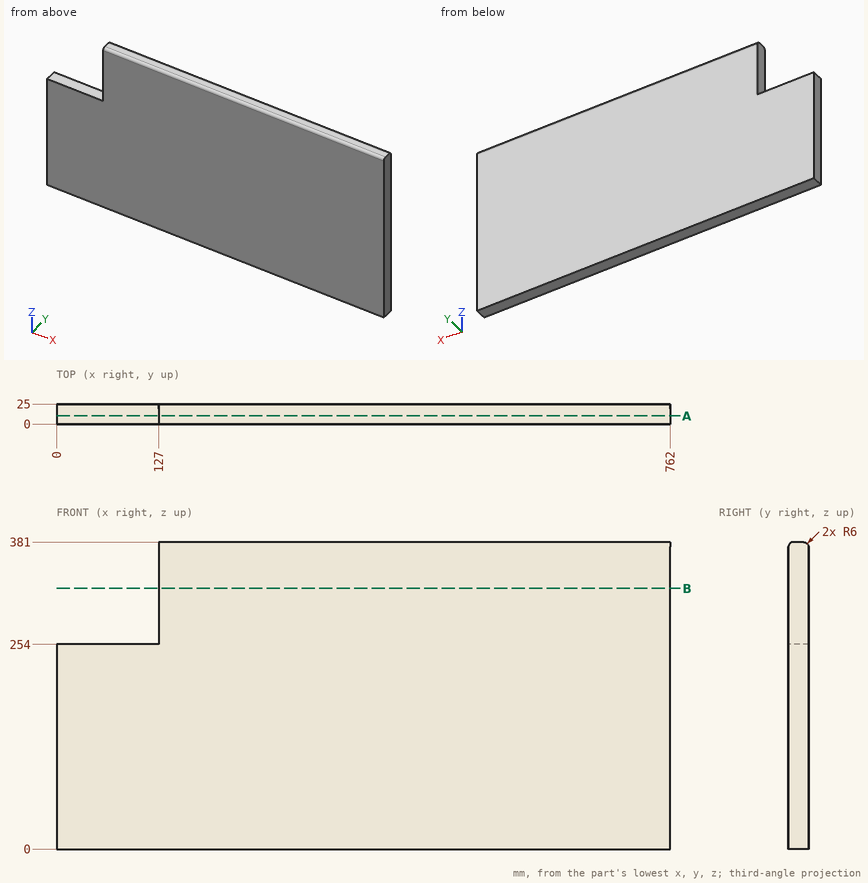
The drawing under review shows one solid part. Ordinate dimensions are in mm from its lowest x, y, z. Give positions to 0.01 mm unless a question says otherwise; leave off trailing zeros. Order: outer loops, then holes, each group sorted by start corner. A loop starts at its lowest first (then second) coordinate and runs counter-clockwise, first axis right, second up. Notation, with made-up numbers: (23.5, -1) -> (53.5, -1) arc R16 cw to (53.5, 10) -> close; hole circle Ø6 at (74.5, -20). An arc over 180 degrees is marked (long way). Write item = value, one per line.
1) Insertion check: pin 1 (12.5 mm diameter, centred on y = 10.5, z = 337.5, fed in from -X). The pin has a flat end and moves straight along its axis. Give the tip position at first contact, or say it passes through.
Findings:
pin_1 = 127
2) We need section B-B, the plane z = 323.5. Give the boundary of the cut face in (x, y), and give its area (3 significant figures).
Findings:
outline = (127, 0) -> (762, 0) -> (762, 25) -> (127, 25) -> close
area = 15,900 mm^2
3) To check wall thickness, follow L1, parallel to Z at x = 65, y = 20.75; L2, parallel to X at y = 21.75, z = 265; L3, parallel to Z at x = 513.5, y = 5.5. State the ranges of each line that lie inside material, in increasing order. Write a range as from..to.
Findings:
L1 = 0..254
L2 = 127..762
L3 = 0..380.98
4) We need section A-A, the plane y = 10.25. Give the boundary of the cut face in (x, z).
Findings:
outline = (0, 0) -> (762, 0) -> (762, 381) -> (127, 381) -> (127, 254) -> (0, 254) -> close
